from build123d import *

# Parameters (mm, degrees)
F0_W           = 101.6
F0_H           = 50.8
F1_DEPTH       = 3.175
F2_R           = 2.54
F4_D           = 3.4
F4_CSINK_D     = 6.72
F4_CSINK_ANGLE = 90


with BuildPart() as f1:
    # F0 (on Top) → F1 (new body)
    with BuildSketch(Plane.XY):
        Rectangle(F0_W, F0_H)
    extrude(amount=-F1_DEPTH)

    # F2
    f2_edges = [f1.edges().sort_by_distance(p)[0] for p in [
        (-50.8, -25.4, -1.5875),
        (50.8, -25.4, -1.5875),
        (50.8, 25.4, -1.5875),
        (-50.8, 25.4, -1.5875),
    ]]
    fillet(f2_edges, radius=F2_R)

    # F4 (through all)
    with Locations(Plane.XY):
        with Locations((-46.355, 20.955), (46.355, 20.955), (46.355, -20.955), (-46.355, -20.955)):
            CounterSinkHole(F4_D / 2, F4_CSINK_D / 2, counter_sink_angle=F4_CSINK_ANGLE)


solid = f1.part
Here's how the part is built. I have some questions about the finished solid (model axes, mm). Round coordinates to 2 decimals unless told otherwise and drop trailing zeros. One line per question, with ' | ' between items. Start each with the question number.
Q1. Please list where these lines run through material, in increasing order: line 1 (X direction, y = -22.5, z = -2.95); line 2 (X direction, y = 21, z = -1.2); line 3 (X direction, y = 23.5, z = -2.35). Write a range as [from, to].
Q2. Will these pins go through, and if not, where does the flat tip stop? pin 1 (2.5 mm diameter, centred on x = 46.355, y = 20.955, fed in from -Z); pin 2 (4 mm diameter, centred on x = -46.355, y = -20.955, fed in from +Z).
Q3. We'd pull the mould along Y, two halves only. Please class faces 1 (the flat face through (50.8, 0, -2)), 2 (the cylindrical face through (-50.076, 24.636, -1.61)), 3 (the cylindrical face through (-45.006, 19.921, -2.428)): +Y half, -Y half, draft (parallel to the pull), parting line (faces both ways), or undercut.
Response values:
1) line 1: x = [-50.8, -47.06], [-45.65, 45.65], [47.06, 50.8] | line 2: x = [-50.8, -48.51], [-44.2, 44.2], [48.51, 50.8] | line 3: x = [-50.72, 50.72]
2) pin 1: passes through | pin 2: stops at z = -1.36
3) face 1: draft | face 2: +Y half | face 3: undercut
